Build history of the part. All positions in model axes, mm. A direction names the side the tool comes from. Coordinates: 2 decimals unless noted, no trailing zeros. Order: outer loops, then holes, each group sorted by start corner. A loop starts at its lowest first (then second) coordinate and runs counter-clockwise, first axis right, second up. Notation, with made-up numbers: (83, 72) - (119, 72) arc R35 ccw to (119, 110) - close; hole circle Ø3 at (60, 14). An arc over 180 degrees is marked (long way). One line per item, written item: value.
from build123d import *

# Parameters (mm, degrees)
BOSS_EXTRUDE1_DEPTH = 1.8


with BuildPart() as part:
    # Sketch1 → Boss-Extrude1 (new, symmetric)
    with BuildSketch(Plane.XY):
        with BuildLine():
            ThreePointArc((-4.21984631, 22.328989928), (-4.242403877, 22.413175911), (-4.25, 22.5))
            Line((-4.25, 22.5), (-1, 22.5))
            Line((-1, 22.5), (6.5, 22.5))
            ThreePointArc((6.5, 22.5), (6.853553391, 22.353553391), (7, 22))
            Line((7, 22), (7, 21.588675135))
            ThreePointArc((7, 21.588675135), (6.933012702, 21.338675135), (6.75, 21.155662433))
            Line((6.75, 21.155662433), (3.25, 19.134936491))
            ThreePointArc((3.25, 19.134936491), (3.066987298, 18.951923789), (3, 18.701923789))
            Line((3, 18.701923789), (3, 0))
            Line((3, 0), (0, 0))
            Line((0, 0), (-3, 0))
            Line((-3, 0), (-3, 18.889326245))
            ThreePointArc((-3, 18.889326245), (-3.007596123, 18.976150334), (-3.03015369, 19.060336317))
            Line((-3.03015369, 19.060336317), (-4.21984631, 22.328989928))
        make_face()
        with BuildLine():
            Line((-4.25, 23.85), (-4.25, 22.5))
            Line((-4.25, 22.5), (-1, 22.5))
            ThreePointArc((-1, 22.5), (-1.353553391, 22.646446609), (-1.5, 23))
            Line((-1.5, 23), (-1.5, 23.85))
            Line((-1.5, 23.85), (-4.25, 23.85))
        make_face()
        with BuildLine():
            Line((-4.25, 25.91183651), (-4.25, 23.85))
            Line((-4.25, 23.85), (-1.5, 23.85))
            Line((-1.5, 23.85), (-1.5, 25.41183651))
            ThreePointArc((-1.5, 25.41183651), (-0.767766953, 27.179603463), (1, 27.91183651))
            Line((1, 27.91183651), (6.5, 27.91183651))
            ThreePointArc((6.5, 27.91183651), (7.855918255, 26.555918255), (6.5, 25.2))
            Line((6.5, 25.2), (0, 25.2))
            Line((0, 25.2), (0, 23.85))
            Line((0, 23.85), (7.413386816, 23.85))
            ThreePointArc((7.413386816, 23.85), (9.318168769, 27.01872909), (6.5, 29.41183651))
            Line((6.5, 29.41183651), (-0.75, 29.41183651))
            ThreePointArc((-0.75, 29.41183651), (-3.224873734, 28.386710244), (-4.25, 25.91183651))
        make_face()
    extrude(amount=BOSS_EXTRUDE1_DEPTH, both=True)

    # Mirror1: part across plane


with BuildPart() as part_1:
    add(part.part)
    add(part.part.mirror(Plane.ZX))


solid = part_1.part
1. 3-axis set-ups, long thin cutter, end or side, ignore diameter. For faces 4 (the face through (1, 0, -1.8)), 5 (the face through (5.024, 20.159, 0.025)), 6 (the face through (-3, 0, 0)), 7 (the face through (3, -25.2, 0)): which of +Z, -Z, +X, -X, +Y, -Y reach the whole face in a straight line?
Values found:
face 4: -Z, +X, -X, +Y, -Y
face 5: +Z, -Z, +X
face 6: +Z, -Z, -X
face 7: +Z, -Z
2. Band-saw the part on A-A, the plane y = -17. Give the cut face in (x, z).
Values found:
outline: (-3, -1.8) - (3, -1.8) - (3, 1.8) - (-3, 1.8) - close
3. Flat gauge pins, fed straight in: P1, Ø1, axis at y = -14.5, z = -0.5, coming from the +X side; P2, Ø0.7, axis at y = -24.5, z = 0, coming from the +X side; P3, Ø1, axis at y = 15, z = -1, coming from the -X side. Where does each tip first touch, or does it go through?
Values found:
P1: stops at x = 3
P2: stops at x = 8.79
P3: stops at x = -3
4. Probe line 1 along Y through (x, z) = (2.5, 1.55); line 2 along Y through (x, z) = (3.25, 0.85); line 3 along Y through (x, z) = (3.5, -1.55). List the from-to ranges inside material, lowest first.
Values found:
line 1: y = -29.41 to -27.91, -25.2 to -23.85, -22.5 to 22.5, 23.85 to 25.2, 27.91 to 29.41
line 2: y = -29.41 to -27.91, -25.2 to -23.85, -22.5 to -19.13, 19.13 to 22.5, 23.85 to 25.2, 27.91 to 29.41
line 3: y = -29.41 to -27.91, -25.2 to -23.85, -22.5 to -19.28, 19.28 to 22.5, 23.85 to 25.2, 27.91 to 29.41
5. Two-plate mould, pull along X, no slides. Class faces 1 (the face through (-1.5, -24, 0)), 2 (the face through (3, 29.412, 0)), 3 (the face through (5.024, -20.159, 0.025)): pulls with the +X half, pulls with the -X half, needs draft (parallel to the pull), parting line crosses it, or undercut.
Values found:
face 1: undercut
face 2: needs draft
face 3: pulls with the +X half
